Geometry: see drawing. Coordinates: mm, zero at the bounding-box minimum. Coordinates: 2 decimals unless noted, no trailing zeros. Order: outer loops, then holes, each group sorted by start corner. A loop starts at its lowest first (then second) coordinate and runs counter-clockwise, first axis right, second up. Notation, with made-up numbers: (87.5, 26.25) - (120.5, 26.25) arc R15 ccw to (120.5, 32.25) - close; hole circle Ø7 at (41.25, 17.5). An arc over 180 degrees is marked (long way). Use a Markdown table: item, result. Add a question column.
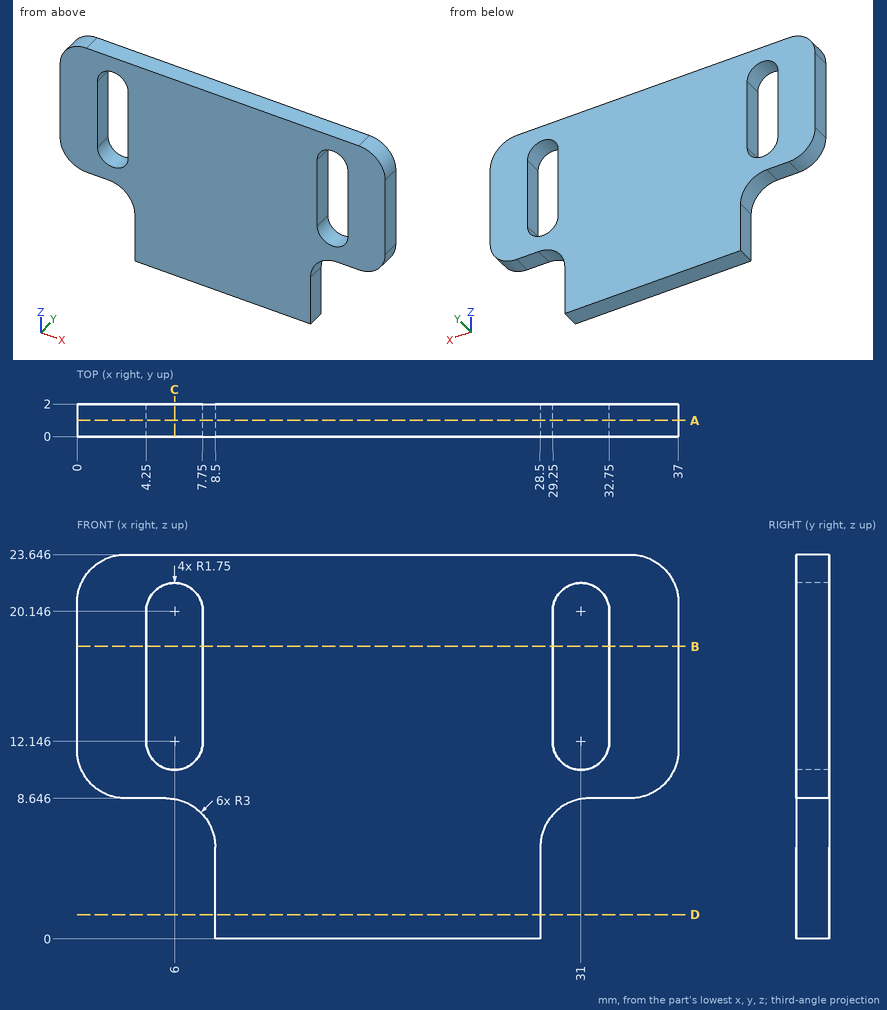
1) Section query B-B (z = 18). Return the cut outline in (x, y), and give its area (3 significant figures).
2) Section query A-A (y = 1). Return the cut outline in (x, z).
3) First-contact query: pin 1 (1 mm diameter, centred on x = 32, y = 1, fed in from -Z); pin 2 (1 mm diameter, centred on y = 1, z = 4, fed in from -X); pin 3 (0.6 mm diameter, centred on y = 1, z = 2, fed in from +X). Flat tips, straight axial feed; report the tip coordinate or a pass-through.
4) Section query D-D (z = 1.5). Return the cut outline in (x, y).
5) Section query C-C (x = 6). Return the cut outline in (y, z).
6) Line query: line 1 (X direction, y = 0.9, z = 20); line 2 (X direction, y = 0.6, z = 2.25); line 3 (Z direction, x = 7, y = 1.25). Output: solid intervals per line, ascending. Write a range as from..to.
From the geometry:
| question | item | result |
|---|---|---|
| 1 | outline | (0, 0) - (4.25, 0) - (4.25, 2) - (0, 2) - close; (7.75, 0) - (29.25, 0) - (29.25, 2) - (7.75, 2) - close; (32.75, 0) - (37, 0) - (37, 2) - (32.75, 2) - close |
| 1 | area | 60.0 mm^2 |
| 2 | outline | (0, 11.65) arc R3 ccw to (3, 8.65) - (5.5, 8.65) arc R3 cw to (8.5, 5.65) - (8.5, 0) - (28.5, 0) - (28.5, 5.65) arc R3 cw to (31.5, 8.65) - (34, 8.65) arc R3 ccw to (37, 11.65) - (37, 20.65) arc R3 ccw to (34, 23.65) - (3, 23.65) arc R3 ccw to (0, 20.65) - close; hole (4.25, 12.15) arc R1.75 ccw to (7.75, 12.15) - (7.75, 20.15) arc R1.75 ccw to (4.25, 20.15) - close; hole (29.25, 12.15) arc R1.75 ccw to (32.75, 12.15) - (32.75, 20.15) arc R1.75 ccw to (29.25, 20.15) - close |
| 3 | pin 1 | stops at z = 8.65 |
| 3 | pin 2 | stops at x = 8.5 |
| 3 | pin 3 | stops at x = 28.5 |
| 4 | outline | (8.5, 0) - (28.5, 0) - (28.5, 2) - (8.5, 2) - close |
| 5 | outline | (0, 8.6) - (2, 8.6) - (2, 10.4) - (0, 10.4) - close; (0, 21.9) - (2, 21.9) - (2, 23.65) - (0, 23.65) - close |
| 6 | line 1 | x = 0..4.25, 7.75..29.25, 32.75..37 |
| 6 | line 2 | x = 8.5..28.5 |
| 6 | line 3 | z = 8.24..10.71, 21.58..23.65 |
